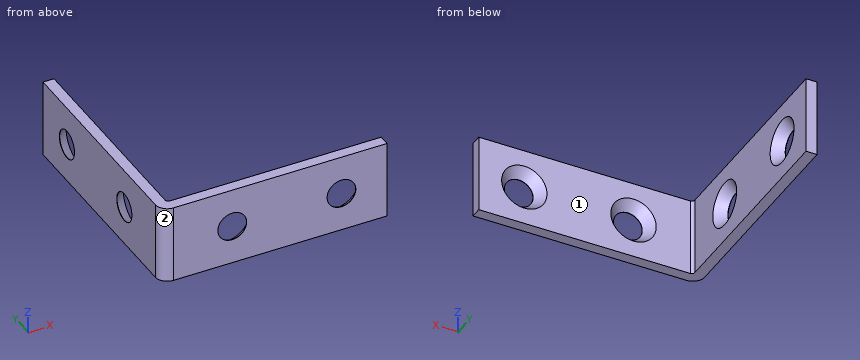
Autodesk Inventor part; units mm, degrees
ref_plane "YZ Plane" through (0, 0, 0) normal (1, 0, 0) x (0, 1, 0)
ref_plane "XZ Plane" through (0, 0, 0) normal (0, 1, 0) x (-1, 0, 0)
ref_plane "XY Plane" through (0, 0, 0) normal (0, 0, 1) x (1, 0, 0)
sketch "Sketch1" plane through (0, 0, 0) normal (0, 0, 1) x (1, 0, 0)
  line L0 (0, 38) -> (1.85, 38)
  line L1 (1.85, 38) -> (1.85, 2.35)
  line L2 (0, 38) -> (0, 2)
  line L3 (38, 0) -> (38, 1.85)
  line L4 (38, 1.85) -> (2.35, 1.85)
  line L5 (38, 0) -> (2, 0)
  arc A0 (1.85, 2.35) -> (2.35, 1.85) centre (2.35, 2.35) ccw
  arc A1 (0, 2) -> (2, 0) centre (2, 2) ccw
  point P0 (0, 0)
  dimension "d0" = 1.85
  dimension "d1" = 1.85
  dimension "d2" = 38
  dimension "d3" = 38
  dimension "d4" = 0.5
  dimension "d5" = 2
extrude "Extrusion1" add sketch "Sketch1" along normal blind 13.2
sketch "Sketch2" plane through (1.85, 2.35, 0) normal (1, 0, 0) x (0, 0, -1)
  circle A0 centre (-6.6, 27.975) radius 2.425
  circle A1 centre (-6.6, 9.575) radius 2.425
  line L0 (0, 35.65) -> (-13.2, 35.65)
  line L1 (-13.2, 0) -> (-13.2, 35.65)
  point P0 (0, -2.35)
  dimension "d8" = 18.4
  dimension "d9" = 4.85
  dimension "d10" = 4.85
  dimension "d11" = 5.25
  dimension "d12" = 13.2
  dimension "d13" = 6.6
  dimension "d14" = 6.6
sketch "Sketch3" plane through (2.35, 1.85, 0) normal (0, 1, 0) x (1, 0, 0)
  circle A0 centre (27.975, -6.6) radius 2.425
  circle A1 centre (9.575, -6.6) radius 2.425
  line L0 (35.65, -13.2) -> (0, -13.2)
  line L1 (35.65, 0) -> (35.65, -13.2)
  point P0 (-2.35, 0)
  dimension "d15" = 18.4
  dimension "d16" = 6.6
  dimension "d17" = 6.6
  dimension "d18" = 4.85
  dimension "d19" = 4.85
  dimension "d20" = 5.25
extrude "Extrusion2" cut sketch "Sketch2" against normal blind 13.2
extrude "Extrusion3" cut sketch "Sketch3" against normal blind 13.2
chamfer "Chamfer1" distance 1.4 distance2 1.8 1 edges at (1.85, 30.325, 9.025) measured on face at (1.85, 23.3649, 1.4152)
chamfer "Chamfer2" distance 1.4 distance2 1.8 1 edges at (9.5, 1.85, 6.6) measured on face at (17.5224, 1.85, 1.3976)
chamfer "Chamfer3" distance 1.4 distance2 1.8 1 edges at (1.85, 11.925, 9.025) measured on face at (1.85, 23.2532, 12.238)
chamfer "Chamfer4" distance 1.4 distance2 1.8 1 edges at (27.9, 1.85, 6.6) measured on face at (17.5787, 1.85, 0.9343)
equation "\"d13\" = 0.5 * d12"
equation "\"d14\" = d13"
equation "\"d17\" = d16"
properties part number "L-Bracket"
The listing builds one solid part. Answer for the finished solid, in the listing's coordinates (mm). Face numbers are marked on the shaded views. A direction names the side the tool comes from. Round coordinates to 2 decimals unless told otherwise and drop trailing zeros. Loops run counter-clockwise (first coordinate to the right, second up) from the corner with the lowest first, then second, coordinate; pieces in that order, holes last.
1) Consider line 1 (X direction, y = 9.5, z = 12.75); line 2 (Y direction, x = 28, z = 5.5). Determine where each line is inside the solid, lowest interval first.
Outcome:
line 1: x = 0 to 1.85
line 2: y = 0 to 0.24
2) A cutting plane is placed at A-A on z = 6.6. Give the number of separate pieces and of enclosed holes in the cut face, plus the area to 3 significant figures.
Outcome:
separate pieces: 5
enclosed holes: 0
area: 90.4 mm2
3) A cutting plane is placed at B-B on z = 1.5. Determine the outline of the cut face in (x, y), plus the area to 3 significant figures.
Outcome:
outline: (0, 2) arc R2 ccw to (2, 0) - (38, 0) - (38, 1.85) - (2.35, 1.85) arc R0.5 cw to (1.85, 2.35) - (1.85, 38) - (0, 38) - close
area: 136 mm2
4) A cutting plane is placed at C-C on x = 21. Determine the outline of the cut face in (y, z).
Outcome:
outline: (0, 0) - (1.85, 0) - (1.85, 13.2) - (0, 13.2) - close
5) For the marked faces 1 and 2, determine the directions among +Z, -Z, +X, -X, +Y, -Y from which every point of the face is accessible in a straight line to the end or side of a thin tool.
Outcome:
face 1: +Z, -Z, +X, +Y
face 2: +Z, -Z, -X, -Y
6) Given P1, Ø6.5, axis at y = 11.925, z = 6.6, coming from the +X side; P2, Ø4, axis at y = 21.5, z = 3.5, coming from the +X side, each flat-ended and moving along its own axis, determine where each tip first touches the part or whether it passes through.
Outcome:
P1: stops at x = 1.11
P2: stops at x = 1.85
